from build123d import *

# Parameters (mm, degrees)
SKETCH1_W           = 92
SKETCH1_H           = 51
BOSS_EXTRUDE1_DEPTH = 2
FILLET1_R           = 6
BOSS_EXTRUDE2_DEPTH = 4
BOSS_EXTRUDE3_DEPTH = 10
CUT_EXTRUDE2_START  = -2
CUT_EXTRUDE2_DEPTH  = 2


with BuildPart() as part:
    # Sketch1 → Boss-Extrude1 (new body)
    with BuildSketch(Plane.XY):
        Rectangle(SKETCH1_W, SKETCH1_H)
    extrude(amount=BOSS_EXTRUDE1_DEPTH)

    # Fillet1
    fillet1_edges = [part.edges().sort_by_distance(p)[0] for p in [
        (46, -25.5, 1),
        (-46, -25.5, 1),
        (-46, 25.5, 1),
        (46, 25.5, 1),
    ]]
    fillet(fillet1_edges, radius=FILLET1_R)

    # Sketch2 → Boss-Extrude2 (add)
    with BuildSketch(Plane.XY.offset(2)):
        with BuildLine():
            Line((-40, -29.5), (40, -29.5))
            ThreePointArc((40, -29.5), (47.071067812, -26.571067812), (50, -19.5))
            Line((50, -19.5), (50, 19.5))
            ThreePointArc((50, 19.5), (47.071067812, 26.571067812), (40, 29.5))
            Line((40, 29.5), (-40, 29.5))
            ThreePointArc((-40, 29.5), (-47.071067812, 26.571067812), (-50, 19.5))
            Line((-50, 19.5), (-50, -19.5))
            ThreePointArc((-50, -19.5), (-47.071067812, -26.571067812), (-40, -29.5))
        make_face()
        with BuildLine():
            Line((-46, 19.5), (-46, -19.5))
            ThreePointArc((-46, -19.5), (-44.242640687, -23.742640687), (-40, -25.5))
            Line((-40, -25.5), (40, -25.5))
            ThreePointArc((40, -25.5), (44.242640687, -23.742640687), (46, -19.5))
            Line((46, -19.5), (46, 19.5))
            ThreePointArc((46, 19.5), (44.242640687, 23.742640687), (40, 25.5))
            Line((40, 25.5), (-40, 25.5))
            ThreePointArc((-40, 25.5), (-44.242640687, 23.742640687), (-46, 19.5))
        make_face(mode=Mode.SUBTRACT)
    extrude(amount=-BOSS_EXTRUDE2_DEPTH)

    # Sketch3 → Boss-Extrude3 (add, symmetric)
    with BuildSketch(Plane(origin=(0, 0, 0), x_dir=(1, 0, 0), z_dir=(0, 1, 0))):
        with BuildLine():
            Line((-41, 7.6), (-41, 0))
            Line((-41, 0), (-38, 0))
            Line((-38, 0), (-38, 10))
            Line((-38, 10), (-39.799999994, 10))
            ThreePointArc((-39.799999994, 10), (-41.141640785, 9.170820396), (-41, 7.6))
        make_face()
        with BuildLine():
            Line((38, 0), (41, 0))
            Line((41, 0), (41, 7.6))
            ThreePointArc((41, 7.6), (41.141640788, 9.17082039), (39.800000006, 10))
            Line((39.800000006, 10), (38, 10))
            Line((38, 10), (38, 0))
        make_face()
    extrude(amount=BOSS_EXTRUDE3_DEPTH, both=True)

    # Sketch4 → Cut-Extrude2 (cut)
    with BuildSketch(Plane(origin=(0, 0, -2), x_dir=(-1, 0, 0), z_dir=(0, 0, -1)).offset(CUT_EXTRUDE2_START)):
        with BuildLine():
            Line((46.1, -19.5), (46.1, 19.5))
            ThreePointArc((46.1, 19.5), (44.313351365, 23.813351365), (40, 25.6))
            Line((40, 25.6), (-40, 25.6))
            ThreePointArc((-40, 25.6), (-44.313351365, 23.813351365), (-46.1, 19.5))
            Line((-46.1, 19.5), (-46.1, -19.5))
            ThreePointArc((-46.1, -19.5), (-44.313351365, -23.813351365), (-40, -25.6))
            Line((-40, -25.6), (40, -25.6))
            ThreePointArc((40, -25.6), (44.313351365, -23.813351365), (46.1, -19.5))
        make_face()
        with BuildLine():
            Line((-40, 25.5), (40, 25.5))
            ThreePointArc((40, 25.5), (44.242640687, 23.742640687), (46, 19.5))
            Line((46, 19.5), (46, -19.5))
            ThreePointArc((46, -19.5), (44.242640687, -23.742640687), (40, -25.5))
            Line((40, -25.5), (-40, -25.5))
            ThreePointArc((-40, -25.5), (-44.242640687, -23.742640687), (-46, -19.5))
            Line((-46, -19.5), (-46, 19.5))
            ThreePointArc((-46, 19.5), (-44.242640687, 23.742640687), (-40, 25.5))
        make_face(mode=Mode.SUBTRACT)
    extrude(amount=CUT_EXTRUDE2_DEPTH, mode=Mode.SUBTRACT)


solid = part.part
Model file for the job. Use its own axes, mm. A direction names the side the tool comes from. Round coordinates to 2 decimals unless told otherwise and drop trailing zeros. Loops run counter-clockwise (first coordinate to the right, second up) from the corner with the lowest first, then second, coordinate; pieces in that order, holes last. Notation, with made-up numbers: (70, -36) - (111, -36) arc R30 ccw to (111, -12) - close; hole circle Ø7 at (40.5, -21). An arc over 180 degrees is marked (long way). Write each question's results on one line, items separated by ' | '.
(1) Mould opens along X. For faces 3 (the cylindrical face through (-44.266, -23.861, -0.986)), 4 (the flat face through (1, 29.5, 0)), 5 (the cylindrical face through (41.15, 0.14, -9.15)), 6 (the flat face through (-50, 0, 0)) say: released by +X, released by -X, zero draft, split by the parting line, or undercut.
Answer below:
face 3: undercut | face 4: zero draft | face 5: released by +X | face 6: released by -X
(2) Wall check: L1, parallel to X at y = -7, z = -0.75; L2, parallel to X at y = -18.5, z = -0.25; L3, parallel to Y at x = -18, z = -0.5. Give the ranges that are in metal, low to high.
Answer below:
L1: x = -50 to -46.1, -41 to -38, 38 to 41, 46.1 to 50 | L2: x = -50 to -46.1, 46.1 to 50 | L3: y = -29.5 to -25.6, 25.6 to 29.5
(3) Saw through at C-C, the plane y = 22.5. List the corners of the cut face in (x, z).
Answer below:
outline: (-49.54, -2) - (-45.31, -2) - (-45.31, 0) - (45.31, 0) - (45.31, -2) - (49.54, -2) - (49.54, 2) - (-49.54, 2) - close
(4) 3-axis set-ups, long thin cutter, end or side, ignore diameter. For faces 1 (the cylindrical face through (47.15, 26.49, 0.03)), 2 (the flat face through (-46.1, 0, -1)): which of +Z, -Z, +X, -X, +Y, -Y reach the whole face in a straight line?
Answer below:
face 1: +Z, -Z, +X, +Y | face 2: -Z
(5) Pin check, flat tips, straight feed: pin 1 (2.5 mm diameter, centred on x = 39.5, z = -6, fed in from +Y); pin 2 (5 mm diameter, centred on y = 1.5, z = -6.5, fed in from -X); pin 3 (1 mm diameter, centred on x = -19, y = -19, fed in from -Z). Stop position of each tip, or through.
Answer below:
pin 1: stops at y = 10 | pin 2: stops at x = -41.3 | pin 3: stops at z = 0
(6) Saw through at D-D, the plane y = -5.5. List the corners of the cut face in (x, z).
Answer below:
outline: (-50, -2) - (-46.1, -2) - (-46.1, 0) - (-41, 0) - (-41, -7.6) arc R1.5 ccw to (-39.8, -10) - (-38, -10) - (-38, 0) - (38, 0) - (38, -10) - (39.8, -10) arc R1.5 ccw to (41, -7.6) - (41, 0) - (46.1, 0) - (46.1, -2) - (50, -2) - (50, 2) - (-50, 2) - close
(7) Saw through at B-B, the plane x = 37. List the corners of the cut face in (y, z).
Answer below:
outline: (-29.5, -2) - (-25.6, -2) - (-25.6, 0) - (25.6, 0) - (25.6, -2) - (29.5, -2) - (29.5, 2) - (-29.5, 2) - close
(8) Saw through at A-A, the plane z = -1. List the corners of the cut face in (x, y), then the cut area to 3 significant figures.
Answer below:
outline: (-50, -19.5) arc R10 ccw to (-40, -29.5) - (40, -29.5) arc R10 ccw to (50, -19.5) - (50, 19.5) arc R10 ccw to (40, 29.5) - (-40, 29.5) arc R10 ccw to (-50, 19.5) - close; (-41, -10) - (-38, -10) - (-38, 10) - (-41, 10) - close; (38, -10) - (41, -10) - (41, 10) - (38, 10) - close; hole (-46.1, -19.5) arc R6.1 ccw to (-40, -25.6) - (40, -25.6) arc R6.1 ccw to (46.1, -19.5) - (46.1, 19.5) arc R6.1 ccw to (40, 25.6) - (-40, 25.6) arc R6.1 ccw to (-46.1, 19.5) - close | area: 1,250 mm^2
